Verification items for the finished model (mm, model axes). Face numbers are marked on the shaded views. A direction names the side the tool comes from. Round coordinates to 2 decimals unless told otherwise and drop trailing zeros. Order: outer loops, then holes, each group sorted by start corner. A loop starts at its lowest first (then second) coordinate and runs counter-clockwise, first axis right, second up. Notation, with made-up numbers: M -8,-0.75 L 34,-0.75 A15 cw 34,15.25 Z; hole C 89.5,66.25 d1. An arc over 180 degrees is marked long. Answer as a JSON object with one key per item and string values. Group by question number.
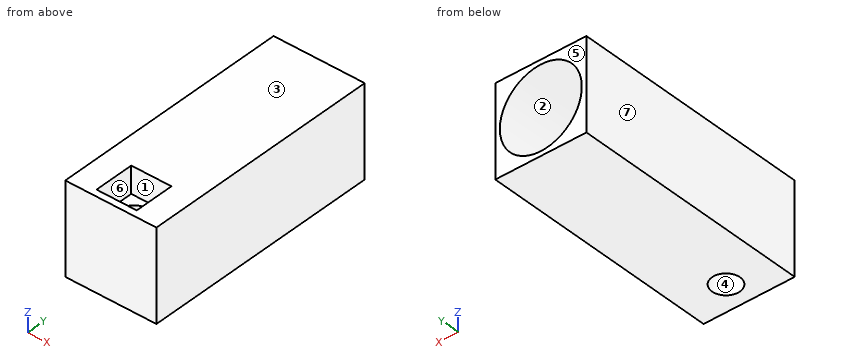
```python
from build123d import *

# Parameters (mm, degrees)
SKETCH1_W           = 21.59
SKETCH1_H           = 21.59
BOSS_EXTRUDE1_DEPTH = 57.15
SKETCH2_W           = 9.525
SKETCH2_H           = 9.525
CUT_EXTRUDE1_DEPTH  = 6.35
SKETCH3_R           = 3.302
CUT_EXTRUDE2_DEPTH  = 16.24
SKETCH4_R           = 9.7155
CUT_EXTRUDE3_DEPTH  = 31.75


with BuildPart() as part:
    # Sketch1 → Boss-Extrude1 (new body)
    with BuildSketch(Plane(origin=(0, 0, 0), x_dir=(1, 0, 0), z_dir=(0, 1, 0))):
        Rectangle(SKETCH1_W, SKETCH1_H)
    extrude(amount=BOSS_EXTRUDE1_DEPTH)

    # Sketch2 → Cut-Extrude1 (cut)
    with BuildSketch(Plane.XY.offset(10.795)):
        with Locations((0, 6.35)):
            Rectangle(SKETCH2_W, SKETCH2_H)
    extrude(amount=-CUT_EXTRUDE1_DEPTH, mode=Mode.SUBTRACT)

    # Sketch3 → Cut-Extrude2 (cut, through all)
    with BuildSketch(Plane.XY.offset(4.445)):
        with Locations((0, 6.35)):
            Circle(SKETCH3_R)
    extrude(amount=-CUT_EXTRUDE2_DEPTH, mode=Mode.SUBTRACT)

    # Sketch4 → Cut-Extrude3 (cut)
    with BuildSketch(Plane(origin=(0, 57.15, 0), x_dir=(1, 0, 0), z_dir=(0, 1, 0))):
        Circle(SKETCH4_R)
    extrude(amount=-CUT_EXTRUDE3_DEPTH, mode=Mode.SUBTRACT)


solid = part.part
```
Q1. Cross-section at D-D, the plane y = 39.5. Record the cut outline in (x, z) (1 decimal).
Q2. Cross-section at A-A, the plane y = 6.35. Record the cut outline in (x, z) (1 decimal), then the cut area to 3 significant figures.
Q3. Thickness scan on line 1 (Z direction, x = 0, y = 34) (1 decimal); line 2 (Y direction, x = 0, z = -5.25). Record the ranges inside material, lowest first. Write a range as from..to.
Q4. Tool access check on the marked faces 1, 2 and 3. Record the directions out of +Z, -Z, +X, -X, +Y, -Y that give a thin tool (end or side, any length) a straight path to the whole face; none if there is none.
Q5. Gauge pin test, flat ends, axial feed: pin 1 Ø1.9 at (x, z) = (2, 6.5) entering from +Y; pin 2 Ø3 at (x, z) = (-2, 9) entering from -Y. Record the tip position at first contact, or that the pin passes through.
Q6. Release check for a two-part mould opening along Y. For the marked faces 4, 5, 6 and 7 record: released by +Y, released by -Y, zero draft, split by the parting line, or undercut.
Conclusion:
{
 "1": {"outline": "M -10.8,-10.8 L 10.8,-10.8 L 10.8,10.8 L -10.8,10.8 Z; hole C 0,0 d19.4"},
 "2": {"outline": "M -10.8,-10.8 L -3.3,-10.8 L -3.3,4.4 L -4.8,4.4 L -4.8,10.8 L -10.8,10.8 Z; M 3.3,-10.8 L 10.8,-10.8 L 10.8,10.8 L 4.8,10.8 L 4.8,4.4 L 3.3,4.4 Z", "area": "305 mm2"},
 "3": {"line 1": "-10.8..-9.7, 9.7..10.8", "line 2": "0..3.05, 9.65..25.4"},
 "4": {"face 1": "+Z", "face 2": "+Y", "face 3": "+Z, +X, -X, +Y, -Y"},
 "5": {"pin 1": "y = 25.4", "pin 2": "y = 0"},
 "6": {"face 4": "undercut", "face 5": "released by +Y", "face 6": "undercut", "face 7": "zero draft"}
}
